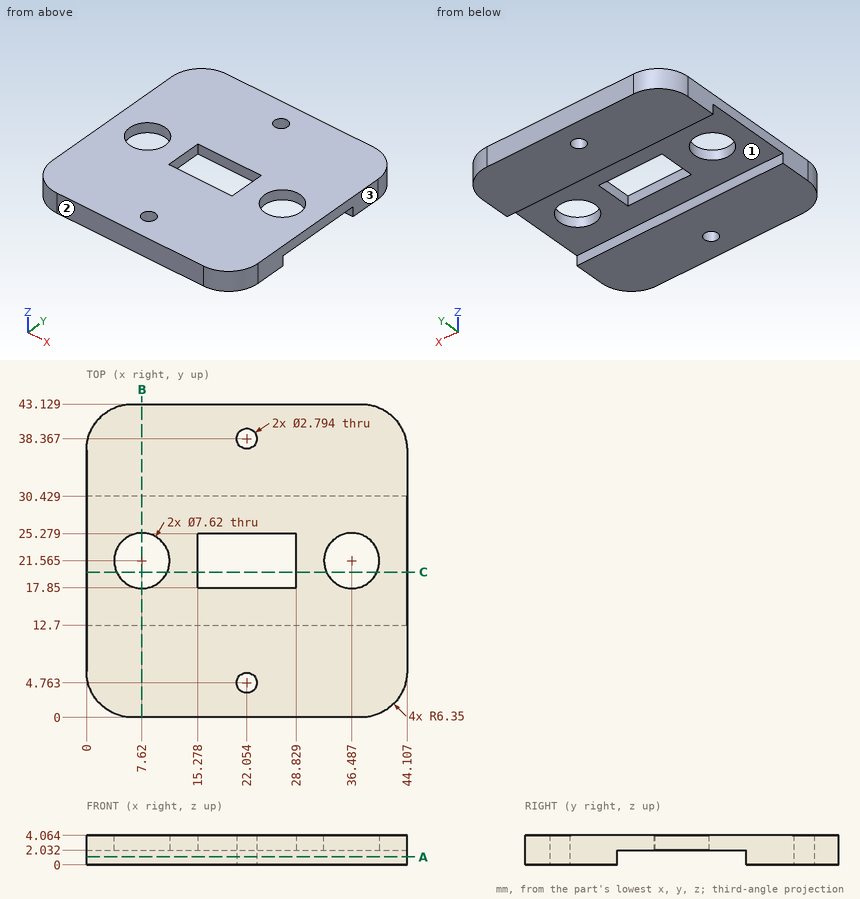
Answer from the drawing. Dimensions are ordinates in mm from the lowest x, y and z of the part. Round coordinates to 2 decimals unless told otherwise and drop trailing zeros. Order: outer loops, then holes, each group sorted by start corner. A loop starts at its lowest first (then second) coordinate and runs counter-clockwise, first axis right, second up. Notation, with made-up numbers: (-8.5, 25.5) - (35.5, 25.5) arc R20 ccw to (35.5, 30.5) - close; hole circle Ø6 at (-34, 79.5). An arc over 180 degrees is marked (long way). Put each result on its own line as item: value. Start each with the question number.
(1) Find section B-B (x = 7.62). Give the vertices of the cut face in (y, z) (1 decimal), plus the area to 3 significant figures.
(2) Determine the mould class of the marked faces 1, 2 and 3 for opening direction Y: released by +Y, released by -Y, zero draft, split by the parting line, or undercut.
(3) Straight lines are drawn through the part: probe 1 along Y at (x, z) = (24, 2.45); probe 2 along Y at (x, z) = (29, 1.95); probe 3 along Z at (x, y) = (42.5, 30) (1 decimal). For each, find the intervals that lie inside material, in ascending order. Write a range as from..to.
(4) Find section A-A (z = 1.1). State how many separate pieces and enclosed holes the cut face has, plus the area to 3 significant figures.
(5) Given P1, Ø3.5, axis at x = 22.05, y = 4.76, coming from the +Z side; P2, Ø14, axis at x = 24, y = 23, coming from the -Z side, each flat-ended and moving along its own axis, determine where each tip first touches the part or whether it passes through.
(6) Find section C-C (y = 20). Give the vertices of the cut face in (x, z) (1 decimal).
Reply:
1. outline: (0, 0) - (12.7, 0) - (12.7, 2) - (17.8, 2) - (17.8, 4.1) - (0, 4.1) - close; (25.4, 2) - (30.4, 2) - (30.4, 0) - (43.1, 0) - (43.1, 4.1) - (25.4, 4.1) - close
1. area: 124 mm^2
2. face 1: undercut
2. face 2: released by -Y
2. face 3: zero draft
3. probe 1: 0..17.85, 25.28..43.13
3. probe 2: 0..12.7, 30.43..43.13
3. probe 3: 2..4.1
4. separate pieces: 2
4. enclosed holes: 2
4. area: 1,070 mm^2
5. P1: z = 4.06
5. P2: z = 2.03
6. outline: (0, 2) - (4.1, 2) - (4.1, 4.1) - (0, 4.1) - close; (11.1, 2) - (15.3, 2) - (15.3, 4.1) - (11.1, 4.1) - close; (28.8, 2) - (33, 2) - (33, 4.1) - (28.8, 4.1) - close; (40, 2) - (44.1, 2) - (44.1, 4.1) - (40, 4.1) - close
